The listing builds one solid part. Answer for the finished solid, in the listing's coordinates (mm). Give positions to 0.01 mm unless a question says otherwise; leave off trailing zeros. Write each loop counter-clockwise with the first axis right and the second up, starting at its lowest first coordinate (ties: lowest second). Pieces come first, ordered by that corner, then holes. Notation, with made-up numbers: M 50.25,10.25 L 81.25,10.25 A13 cw 81.25,17.25 Z; hole C -25,44.25 d7. An arc over 180 degrees is marked long. Return JSON: item names as keys, results as strings.
from build123d import *

# Parameters (mm, degrees)
SKETCH1_W                               = 15
SKETCH1_H                               = 37.5
BOSS_EXTRUDE1_DEPTH                     = 4.5
SKETCH2_R                               = 5
CUT_EXTRUDE1_DEPTH                      = 5
CUT_EXTRUDE1_TAPER                      = 10
CUT_EXTRUDE1_OTHER_WAY_DEPTH            = 39.568121551
OFFSET_TO_ACCOUNT_FOR_BASE_THICKNESS_BY = 5
CHAMFER1_SIZE                           = 1.25


# Read off the part's stored shape, not the designer's step: Offset for 3D print
with BuildPart() as part:
    # Sketch1 → Boss-Extrude1 (new body)
    with BuildSketch(Plane(origin=(0, 0, 0), x_dir=(0, 0, -1), z_dir=(1, 0, 0))):
        with Locations((0, 18.75)):
            Rectangle(SKETCH1_W, SKETCH1_H)
    extrude(amount=-BOSS_EXTRUDE1_DEPTH)

    # Sketch2 → Cut-Extrude1 (cut)
    with BuildSketch(Plane(origin=(-5, 0, 0), x_dir=(0, 0, -1), z_dir=(1, 0, 0))):
        with Locations((0, 30)):
            Circle(SKETCH2_R)
    extrude(amount=CUT_EXTRUDE1_DEPTH, taper=CUT_EXTRUDE1_TAPER, mode=Mode.SUBTRACT)

    # Sketch2 → Cut-Extrude1 other way (cut)
    with BuildSketch(Plane(origin=(-5, 0, 0), x_dir=(0, 0, -1), z_dir=(1, 0, 0))):
        with Locations((0, 30)):
            Circle(SKETCH2_R)
    extrude(amount=-CUT_EXTRUDE1_OTHER_WAY_DEPTH, mode=Mode.SUBTRACT)

    # Offset to account for Base Thickness: a face moved outward by 5.0
    extrude(part.faces().sort_by_distance((-2.25, 0, 0))[0], amount=OFFSET_TO_ACCOUNT_FOR_BASE_THICKNESS_BY, dir=(0, -1, 0))

    # Chamfer1
    chamfer1_edges = [part.edges().sort_by_distance(p)[0] for p in [
        (-2.25, -5, -7.5),
        (-2.25, -5, 7.5),
        (-2.25, 37.5, 7.5),
        (-2.25, 37.5, -7.5),
    ]]
    chamfer(chamfer1_edges, length=CHAMFER1_SIZE)

    # Offset for 3D print outline → Offset for 3D print (revolve, cut)
    with BuildSketch(Plane(origin=(0, 30, 0), x_dir=(0, 1, 0), z_dir=(0, 0, -1))):
        Polygon((4.118365096, 0), (4.91183651, -4.5), (5.064150501, -4.5), (4.270679088, 0), align=None)
    revolve(axis=Axis((0, 30, 0), (1, 0, 0)), mode=Mode.SUBTRACT)


solid = part.part
Item 1: Determine the mould class of faces 1 (the flat face through (0, 17, 0)), 2 (the flat face through (-2.22, -4.38, 6.87)), 3 (the conical face through (-1.219, 34.278, 1.347)) for opening direction Y: +Y half, -Y half, draft (parallel to the pull), parting line (faces both ways), or undercut.
Geometry results:
{"face 1": "draft", "face 2": "-Y half", "face 3": "undercut"}
Item 2: A cutting plane is placed at C-C, the plane x = -1.05. Write down the section's boundary in (y, z).
Geometry results:
{"outline": "M -5,-6.25 L -3.75,-7.5 L 36.25,-7.5 L 37.5,-6.25 L 37.5,6.25 L 36.25,7.5 L -3.75,7.5 L -5,6.25 Z; hole C 30,0 d8.91"}
Item 3: A cutting plane is placed at D-D, the plane x = -3.7. Write down the section's boundary in (y, z).
Geometry results:
{"outline": "M -5,-6.25 L -3.75,-7.5 L 36.25,-7.5 L 37.5,-6.25 L 37.5,6.25 L 36.25,7.5 L -3.75,7.5 L -5,6.25 Z; hole C 30,0 d9.85"}
Item 4: A cutting plane is placed at A-A, the plane z = 0. Write down the section's boundary in (x, y), plus the area to 3 significant figures.
Geometry results:
{"outline": "M -4.5,-5 L 0,-5 L 0,25.73 L -4.5,24.94 Z; M -4.5,35.06 L 0,34.27 L 0,37.5 L -4.5,37.5 Z", "area": "149 mm2"}
Item 5: A cutting plane is placed at B-B, the plane y = 30. Write down the section's boundary in (x, z), plus the area to 3 significant figures.
Geometry results:
{"outline": "M -4.5,-7.5 L 0,-7.5 L 0,-4.27 L -4.5,-5.06 Z; M -4.5,5.06 L 0,4.27 L 0,7.5 L -4.5,7.5 Z", "area": "25.5 mm2"}
Item 6: Find the intervals of material crossed by line 1 (Y direction, x = -1.7, z = -2.25); line 2 (Y direction, x = -2.55, z = 4); line 3 (Z direction, x = -0.55, y = 33), in increasing order.
Geometry results:
{"line 1": "y = -5 to 26.02, 33.98 to 37.5", "line 2": "y = -5 to 27.49, 32.51 to 37.5", "line 3": "z = -7.5 to -3.17, 3.17 to 7.5"}
